```python
from build123d import *

# Parameters (mm, degrees)
SKETCH_W        = 40
SKETCH_H        = 95
PAD_DEPTH       = 9
SKETCH001_W     = 40
SKETCH001_H     = 50
POCKET_DEPTH    = 4
SKETCH002_R     = 11
PAD001_DEPTH    = 3
SKETCH003_R     = 1.6
POCKET001_DEPTH = 8
SKETCH004_R     = 11
SKETCH004_R_2   = 1.6
POCKET002_DEPTH = 10
FILLET_R        = 6


with BuildPart() as part:
    # Sketch → Pad (new body)
    with BuildSketch(Plane.YZ):
        with Locations((20, 47.5)):
            Rectangle(SKETCH_W, SKETCH_H)
    extrude(amount=PAD_DEPTH)

    # Sketch001 (on Face6 of Pad) → Pocket (cut)
    with BuildSketch(Plane.YZ.offset(9)):
        with Locations((20, 25)):
            Rectangle(SKETCH001_W, SKETCH001_H)
    extrude(amount=-POCKET_DEPTH, mode=Mode.SUBTRACT)

    # Sketch002 (on Face4 of Pocket) → Pad001 (join)
    with BuildSketch(Plane.YZ.offset(5)):
        with Locations((20, 20)):
            Circle(SKETCH002_R)
    extrude(amount=PAD001_DEPTH)

    # Sketch003 (on Face4 of Pad001) → Pocket001 (cut)
    with BuildSketch(Plane.YZ.offset(5)):
        with Locations((4.5, 35.5)):
            Circle(SKETCH003_R)
        with Locations((35.5, 35.5)):
            Circle(SKETCH003_R)
        with Locations((35.5, 4.5)):
            Circle(SKETCH003_R)
        with Locations((4.5, 4.5)):
            Circle(SKETCH003_R)
    extrude(amount=-POCKET001_DEPTH, mode=Mode.SUBTRACT)

    # Sketch004 (on Face11 of Pocket001) → Pocket002 (cut)
    with BuildSketch(Plane.YZ.offset(9)):
        with Locations((20, 72)):
            Circle(SKETCH004_R)
        with Locations((4.5, 87.5)):
            Circle(SKETCH004_R_2)
        with Locations((35.5, 87.5)):
            Circle(SKETCH004_R_2)
        with Locations((35.5, 56.5)):
            Circle(SKETCH004_R_2)
        with Locations((4.5, 56.5)):
            Circle(SKETCH004_R_2)
    extrude(amount=-POCKET002_DEPTH, mode=Mode.SUBTRACT)

    # Fillet
    fillet_edges = [part.edges().sort_by_distance(p)[0] for p in [
        (4.5, 0, 95),
        (4.5, 40, 95),
        (2.5, 40, 0),
        (2.5, 0, 0),
    ]]
    fillet(fillet_edges, radius=FILLET_R)


solid = part.part
```
Work out the finished part from the listing and answer in its coordinate system (mm). A direction names the side the tool comes from. Coordinates: 2 decimals unless noted, no trailing zeros. Write each loop counter-clockwise with the first axis right and the second up, starting at its lowest first coordinate (ties: lowest second). Pieces come first, ordered by that corner, then holes.
Q1. A cutting plane is placed at B-B, the plane z = 72. Give the vertices of the cut face in (x, y), then the cut area to 3 significant figures.
Q2. A cutting plane is placed at C-C, the plane y = 20. Give the vertices of the cut face in (x, z), then the cut area to 3 significant figures.
Q3. A cutting plane is placed at D-D, the plane z = 56.5. Give the vertices of the cut face in (x, y).
Q4. Determine the mould class of faces 1 (the face through (3, 40, 56)), 2 (the face through (4.56, 5.36, 57.85)), 3 (the face through (4.563, 1.711, 93.196)) for opening direction Z: released by +Z, released by -Z, zero draft, split by the parting line, or undercut.
Q5. Each of these flat-tipped pins is pushed along its axis until it touches: pin 1 Ø5 at (y, z) = (35.5, 35.5) entering from +X; pin 2 Ø2.5 at (y, z) = (35.5, 87.5) entering from +X; pin 3 Ø2 at (x, y) = (6.5, 10) entering from -Z; pin 4 Ø24 at (y, z) = (24, 23.5) entering from +X. Where does it stop, or does it pass through?
Q6. A cutting plane is placed at A-A, the plane x = 7. Give the vertices of the cut face in (y, z).
Q7. Which of the six approach directions +Z, -Z, +X, -X, +Y, -Y give full straight-line access (tool end or side, diameter ignored) to faces 4 (the face through (4.563, 4.292, 89.086)), 5 (the face through (7, 20, 50)), 6 (the face through (8, 20, 20)), 7 (the face through (6.479, 30.161, 15.787))?
Q8. Find the intervals of material crossed by line 1 (Y direction, x = 5.75, z = 87.5); line 2 (Z direction, x = 2.25, y = 4.5); line 3 (X direction, y = 9, z = 39), in increasing order.
Findings below:
1. outline: (0, 0) - (9, 0) - (9, 9) - (0, 9) - close; (0, 31) - (9, 31) - (9, 40) - (0, 40) - close
1. area: 162 mm2
2. outline: (0, 0) - (5, 0) - (5, 9) - (8, 9) - (8, 31) - (5, 31) - (5, 50) - (9, 50) - (9, 61) - (0, 61) - close; (0, 83) - (9, 83) - (9, 95) - (0, 95) - close
2. area: 523 mm2
3. outline: (0, 0) - (9, 0) - (9, 2.9) - (0, 2.9) - close; (0, 6.1) - (9, 6.1) - (9, 33.9) - (0, 33.9) - close; (0, 37.1) - (9, 37.1) - (9, 40) - (0, 40) - close
4. face 1: zero draft
4. face 2: undercut
4. face 3: released by +Z
5. pin 1: stops at x = 5
5. pin 2: passes through
5. pin 3: stops at z = 13.68
5. pin 4: stops at x = 8
6. outline: (0, 50) - (40, 50) - (40, 89) arc R6 ccw to (34, 95) - (6, 95) arc R6 ccw to (0, 89) - close; circle Ø22 at (20, 20); hole circle Ø3.2 at (4.5, 56.5); hole circle Ø3.2 at (4.5, 87.5); hole circle Ø22 at (20, 72); hole circle Ø3.2 at (35.5, 56.5); hole circle Ø3.2 at (35.5, 87.5)
7. face 4: +X, -X
7. face 5: +X, +Y, -Y
7. face 6: -Z, +X, +Y, -Y
7. face 7: +X
8. line 1: y = 0 to 2.9, 6.1 to 33.9, 37.1 to 40
8. line 2: z = 0.19 to 2.9, 6.1 to 33.9, 37.1 to 54.9, 58.1 to 85.9, 89.1 to 94.81
8. line 3: x = 0 to 5
